Read the model definition and answer for the solid it produces. Units are mm, in the model's axes. Give positions to 0.01 mm unless a question says otherwise; leave off trailing zeros. Order: outer loops, then holes, each group sorted by start corner. A loop starts at its lowest first (then second) coordinate and runs counter-clockwise, first axis right, second up. Notation, with made-up numbers: (-13.75, 33) - (6.25, 33) arc R21 ccw to (6.25, 52) - close; hole circle Ø4 at (36.5, -27). An arc over 180 degrees is marked (long way). Return JSON: item names as keys, results as strings.
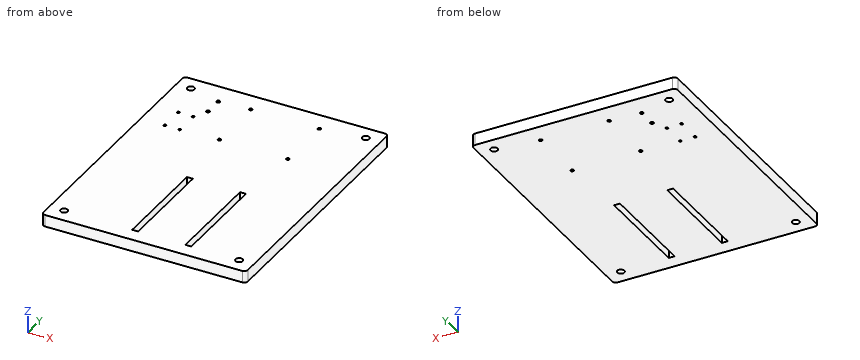
```python
from build123d import *

# Parameters (mm, degrees)
CROQUIS1_R              = 3
CROQUIS1_W              = 5
CROQUIS1_H              = 85.41873638
CROQUIS1_W_2            = 23.862
CROQUIS1_H_2            = 25
CROQUIS1_W_3            = 15
CROQUIS1_H_3            = 20
CROQUIS1_R_2            = 1.5
CROQUIS1_R_3            = 1.1
CROQUIS1_R_4            = 1.35
SALIENTE_EXTRUIR1_DEPTH = 10


with BuildPart() as part:
    # Croquis1 → Saliente-Extruir1 (new body)
    with BuildSketch(Plane.XY):
        with BuildLine():
            ThreePointArc((83.492, 111.366), (85.613320344, 110.487320344), (86.492, 108.366))
            Line((86.492, 108.366), (86.492, -108.366))
            ThreePointArc((86.492, -108.366), (85.613320344, -110.487320344), (83.492, -111.366))
            Line((83.492, -111.366), (-83.492, -111.366))
            ThreePointArc((-83.492, -111.366), (-85.613320344, -110.487320344), (-86.492, -108.366))
            Line((-86.492, -108.366), (-86.492, 108.366))
            ThreePointArc((-86.492, 108.366), (-85.613320344, 110.487320344), (-83.492, 111.366))
            Line((-83.492, 111.366), (83.492, 111.366))
        make_face()
        with Locations((74.136, 98.992)):
            Circle(CROQUIS1_R, mode=Mode.SUBTRACT)
        with Locations((-74.136, 98.992)):
            Circle(CROQUIS1_R, mode=Mode.SUBTRACT)
        with Locations((74.136, -98.992)):
            Circle(CROQUIS1_R, mode=Mode.SUBTRACT)
        with Locations((-74.136, -98.992)):
            Circle(CROQUIS1_R, mode=Mode.SUBTRACT)
        with BuildLine():
            ThreePointArc((55.881809493, 42.260900296), (58.356683228, 43.286026562), (59.381809493, 45.760900296))
            Line((59.381809493, 45.760900296), (59.381809493, 94.012))
            ThreePointArc((59.381809493, 94.012), (58.356683228, 96.486873734), (55.881809493, 97.512))
            Line((55.881809493, 97.512), (-22.118190507, 97.512))
            ThreePointArc((-22.118190507, 97.512), (-24.593064241, 96.486873734), (-25.618190507, 94.012))
            Line((-25.618190507, 94.012), (-25.618190507, 45.760900296))
            ThreePointArc((-25.618190507, 45.760900296), (-24.593064241, 43.286026562), (-22.118190507, 42.260900296))
            Line((-22.118190507, 42.260900296), (55.881809493, 42.260900296))
        make_face(mode=Mode.SUBTRACT)
        with Locations((31.008, -56.19736819)):
            Rectangle(CROQUIS1_W, CROQUIS1_H, mode=Mode.SUBTRACT)
        with Locations((-13.992, -56.19736819)):
            Rectangle(CROQUIS1_W, CROQUIS1_H, mode=Mode.SUBTRACT)
        with Locations((-56.067, 54.012)):
            Rectangle(CROQUIS1_W_2, CROQUIS1_H_2, mode=Mode.SUBTRACT)
        with Locations((-52.84846771, 84.244)):
            Rectangle(CROQUIS1_W_3, CROQUIS1_H_3, mode=Mode.SUBTRACT)
        with Locations((-52.84846771, 84.244)):
            Rectangle(CROQUIS1_W_3, CROQUIS1_H_3)
        with Locations((-47.26410382, 92.23269661)):
            Circle(CROQUIS1_R_2, mode=Mode.SUBTRACT)
        with Locations((-47.26410382, 76.25530339)):
            Circle(CROQUIS1_R_2, mode=Mode.SUBTRACT)
        with Locations((-56.067, 54.012)):
            Rectangle(CROQUIS1_W_2, CROQUIS1_H_2)
        with Locations((-53.498, 64.512)):
            Circle(CROQUIS1_R_3, mode=Mode.SUBTRACT)
        with Locations((-53.498, 43.512)):
            Circle(CROQUIS1_R_3, mode=Mode.SUBTRACT)
        with Locations((-65.998, 43.512)):
            Circle(CROQUIS1_R_3, mode=Mode.SUBTRACT)
        with Locations((-65.998, 64.512)):
            Circle(CROQUIS1_R_3, mode=Mode.SUBTRACT)
        with BuildLine():
            Line((-22.118190507, 42.260900296), (55.881809493, 42.260900296))
            ThreePointArc((55.881809493, 42.260900296), (58.356683228, 43.286026562), (59.381809493, 45.760900296))
            Line((59.381809493, 45.760900296), (59.381809493, 94.012))
            ThreePointArc((59.381809493, 94.012), (58.356683228, 96.486873734), (55.881809493, 97.512))
            Line((55.881809493, 97.512), (-22.118190507, 97.512))
            ThreePointArc((-22.118190507, 97.512), (-24.593064241, 96.486873734), (-25.618190507, 94.012))
            Line((-25.618190507, 94.012), (-25.618190507, 45.760900296))
            ThreePointArc((-25.618190507, 45.760900296), (-24.593064241, 43.286026562), (-22.118190507, 42.260900296))
        make_face()
        with Locations((-20.636, 94.012)):
            Circle(CROQUIS1_R_4, mode=Mode.SUBTRACT)
        with Locations((37.364, 94.012)):
            Circle(CROQUIS1_R_4, mode=Mode.SUBTRACT)
        with Locations((37.364, 45.012)):
            Circle(CROQUIS1_R_4, mode=Mode.SUBTRACT)
        with Locations((-20.636, 45.012)):
            Circle(CROQUIS1_R_4, mode=Mode.SUBTRACT)
    extrude(amount=SALIENTE_EXTRUIR1_DEPTH)


solid = part.part
```
Q1. A cutting plane is placed at A-A (y = -92.5). Write down the section's boundary in (x, z).
Values:
{"outline": "(-86.49, 0) - (-16.49, 0) - (-16.49, 10) - (-86.49, 10) - close; (-11.49, 0) - (28.51, 0) - (28.51, 10) - (-11.49, 10) - close; (33.51, 0) - (86.49, 0) - (86.49, 10) - (33.51, 10) - close"}
Q2. A cutting plane is placed at B-B (z = 7). Give the number of separate pieces and of enclosed holes in the cut face, and give its area (3 significant figures).
Values:
{"separate pieces": "1", "enclosed holes": "16", "area": "37,500 mm²"}
Q3. Consider L1, parallel to X at y = -28.5, z = 3.75; L2, parallel to X at y = -99.5, z = 4; L3, parallel to Y at x = -75, z = 3.5. Determine where each line is inside the solid, lowest interval first.
Values:
{"L1": "x = -86.49 to -16.49, -11.49 to 28.51, 33.51 to 86.49", "L2": "x = -86.49 to -77.09, -71.18 to 71.18, 77.09 to 86.49", "L3": "y = -111.37 to -101.86, -96.12 to 96.12, 101.86 to 111.37"}
Q4. Given pin 1 (3 mm diameter, centred on x = -20.636, y = 94.012, fed in from -Z), flat-ended and moving along its own axis, determine where the tip first touches the part or whether it passes through.
Values:
{"pin 1": "stops at z = 0"}
